Design review of the part shown in the three views and the two pictorial views. Dimensions are in mm from the part's minimum x, y and z. A direction names the side the tool comes from. Coordinates: 2 decimals unless noted, no trailing zeros. Loops run counter-clockwise (first coordinate to the right, second up) from the corner with the lowest first, then second, coordinate; pieces in that order, holes last. Notation, with made-up numbers: M -2,33.25 L 5,33.25 A24 ccw 5,69.25 Z; hole C 13.25,13.25 d2. An arc over 180 degrees is marked long. Write item = value, one per line. Start each with the question number.
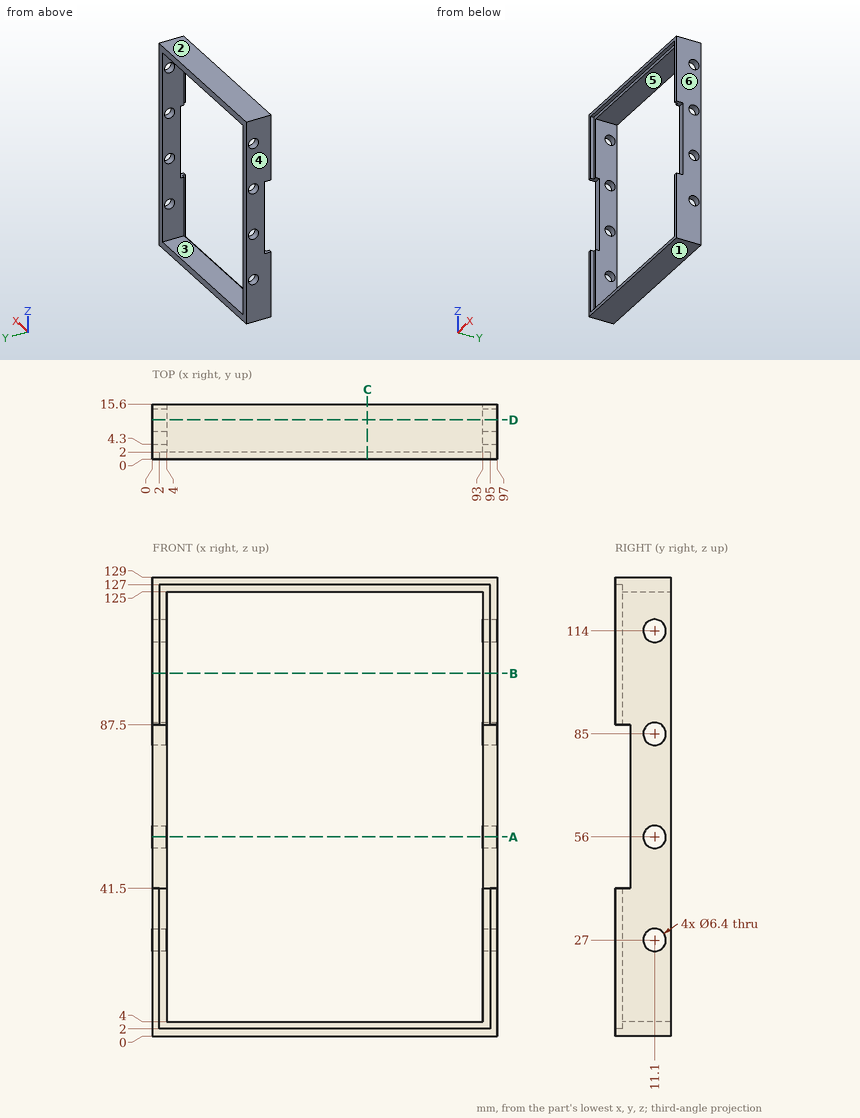
(1) To check wall thickness, follow L1, parallel to Z at x = 82.5, y = 4.25; L2, parallel to X at y = 7.5, z = 16; L3, parallel to Y at x = 95.4, z = 56. State the ranges of each line that lie inside material, in increasing order.
(2) Tool access review of the marked faces 5 and 6: name each direction out of +Z, -Z, +X, -X, +Y, -Y from which nothing blocks a thin tool from reaching the whole face with its end or side.
(3) Take a section at D-D (y = 11.1). Give the number of separate pieces and of enclosed holes in the cut face, plus the area to 3 significant figures.
(4) Take a section at B-B (z = 102). State the section outline as (x, y) points.
(5) Mouldability with a two-part tool opening along Z and no side actions: class the marked faces 1, 2, 3 and 4 as +Z half, -Z half, draft (parallel to the pull), parting line (faces both ways), or undercut.
(6) Take a section at A-A (z = 56). State the section outline as (x, y) points.
(7) Take a section at C-C (x = 60.5). State the section outline as (y, z) points, plus the area to 3 significant figures.
(8) Insertion check: pin 1 (1.2 mm diameter, centred on x = 94.5, z = 64, fed in from -Y). The pin has a flat end and moves straight along its axis. Give the tip position at first contact, or say it passes through.
Results list:
q1.L1 = 0 to 4, 125 to 129
q1.L2 = 0 to 4, 93 to 97
q1.L3 = 4.3 to 7.9, 14.3 to 15.6
q2.face_5 = +Y, -Y
q2.face_6 = +Z, -Z, +X, +Y, -Y
q3.separate_pieces = 8
q3.enclosed_holes = 0
q3.area = 1,540 mm^2
q4.outline = M 0,0 L 2,0 L 2,2 L 4,2 L 4,15.6 L 0,15.6 Z; M 93,2 L 95,2 L 95,0 L 97,0 L 97,15.6 L 93,15.6 Z
q5.face_1 = -Z half
q5.face_2 = +Z half
q5.face_3 = undercut
q5.face_4 = draft
q6.outline = M 0,4.3 L 4,4.3 L 4,7.9 L 0,7.9 Z; M 0,14.3 L 4,14.3 L 4,15.6 L 0,15.6 Z; M 93,4.3 L 97,4.3 L 97,7.9 L 93,7.9 Z; M 93,14.3 L 97,14.3 L 97,15.6 L 93,15.6 Z
q7.outline = M 0,0 L 15.6,0 L 15.6,4 L 2,4 L 2,2 L 0,2 Z; M 0,127 L 2,127 L 2,125 L 15.6,125 L 15.6,129 L 0,129 Z
q7.area = 117 mm^2
q8.pin_1 = 4.3
